from build123d import *

# Parameters (mm, degrees)
F0_W     = 5
F0_H     = 1
F1_DEPTH = 4
F2_DEPTH = 1
F3_SIZE  = 0.99999


# Not quite as in the source:
# - a fillet or chamfer is up to 0.001 mm smaller than in the source, because OpenCascade refuses the exact size


with BuildPart() as f1:
    # F0 (on Top) → F1 (new body)
    with BuildSketch(Plane.XY):
        with Locations((0, 29.5871215252)):
            Rectangle(F0_W, F0_H)
    extrude(amount=F1_DEPTH)

    # F0 (on Top) → F2 (join)
    with BuildSketch(Plane.XY):
        with BuildLine():
            Line((-50, 0), (50, 0))
            ThreePointArc((50, 0), (0, 32.0871215252), (-50, 0))
        make_face()
        with Locations((0, 29.5871215252)):
            Rectangle(F0_W, F0_H, mode=Mode.SUBTRACT)
    extrude(amount=F2_DEPTH)

    # F3 (size 1 in the source; OpenCascade refuses exactly that, so slightly less here)
    f3_edges = [f1.edges().sort_by_distance(p)[0] for p in [
        (0, 32.087122, 0),
        (0, 0, 0),
    ]]
    chamfer(f3_edges, length=F3_SIZE)


solid = f1.part
The listing builds one solid part. Answer for the finished solid, in the listing's coordinates (mm). A direction names the side the tool comes from. Give positions to 0.01 mm unless a question says otherwise; leave off trailing zeros. Write each loop counter-clockwise with the first axis right and the second up, starting at its lowest first coordinate (ties: lowest second). Pieces come first, ordered by that corner, then holes.
Item 1: Which of the six approach directions +Z, -Z, +X, -X, +Y, -Y give full straight-line access (tool end or side, diameter ignored) to faces 1 (the flat face through (0, 30.087, 2)), 2 (the flat face through (-1, 13, 0)), 3 (the flat face through (0, 29.087, 2))?
Item 2: Find the intervals of material crossed by line 1 along Z through (x, y) = (19, 24.5); line 2 along Y through (x, z) = (-14.5, 0.5); line 3 along X through (y, z) = (21, 0.65), in increasing order.
Item 3: Section A-A, the plane z = 2.05 is taken. Write down the section's boundary in (x, y), plus the area to 3 significant figures.
Item 4: Flat-ended cylindrical pins translate along their axes: P1, Ø0.5, axis at y = 29.5, z = 2.5, coming from the -X side; P2, Ø8, axis at x = -7.5, y = 18, coming from the -Z side; P3, Ø2, axis at x = -13.5, z = 0.5, coming from the -Y side; P4, Ø1.5, axis at y = 23.5, z = 0.5, coming from the -X side. Find the tip coordinate at first contact, or state that the pin passes through.
Completed:
1. face 1: +Z, +X, -X, +Y
1. face 2: -Z, +X, -X, +Y, -Y
1. face 3: +Z, +X, -X, -Y
2. line 1: z = 0 to 1
2. line 2: y = 0.5 to 29.62
2. line 3: x = -32.53 to 32.53
3. outline: (-2.5, 29.09) - (2.5, 29.09) - (2.5, 30.09) - (-2.5, 30.09) - close
3. area: 5.00 mm2
4. P1: stops at x = -2.5
4. P2: stops at z = 0
4. P3: stops at y = 0
4. P4: stops at x = -30.37
